```python
from build123d import *

# Parameters (mm, degrees)
SKETCH007_R   = 1.5
SKETCH007_W   = 93.5
SKETCH007_H   = 73
PAD004_DEPTH  = 1.5
SKETCH008_W   = 96.5
SKETCH008_H   = 76
SKETCH008_W_2 = 93.5
SKETCH008_H_2 = 73
PAD005_DEPTH  = 10
FILLET005_R   = 1


with BuildPart() as part:
    # Sketch007 → Pad004 (new body)
    with BuildSketch(Plane.XY):
        with BuildLine():
            Line((-48.25, -33), (-48.25, 33))
            Line((-48.25, 33), (-52.492641, 37.242641))
            ThreePointArc((-47.492641, 42.242641), (-52.492641, 42.242641), (-52.492641, 37.242641))
            Line((-43.25, 38), (-47.492641, 42.242641))
            Line((-43.25, 38), (43.25, 38))
            Line((43.25, 38), (47.492641, 42.242641))
            ThreePointArc((52.492641, 37.242641), (52.492641, 42.242641), (47.492641, 42.242641))
            Line((48.25, 33), (52.492641, 37.242641))
            Line((48.25, 33), (48.25, -33))
            Line((48.25, -33), (52.492641, -37.242641))
            ThreePointArc((47.492641, -42.242641), (52.492641, -42.242641), (52.492641, -37.242641))
            Line((43.25, -38), (47.492641, -42.242641))
            Line((43.25, -38), (-43.25, -38))
            Line((-43.25, -38), (-47.492641, -42.242641))
            ThreePointArc((-52.492641, -37.242641), (-52.492641, -42.242641), (-47.492641, -42.242641))
            Line((-48.25, -33), (-52.492641, -37.242641))
        make_face()
        with Locations((49.992641, -39.742641)):
            Circle(SKETCH007_R, mode=Mode.SUBTRACT)
        with Locations((-49.992641, -39.742641)):
            Circle(SKETCH007_R, mode=Mode.SUBTRACT)
        with Locations((-49.992641, 39.742641)):
            Circle(SKETCH007_R, mode=Mode.SUBTRACT)
        with Locations((49.992641, 39.742641)):
            Circle(SKETCH007_R, mode=Mode.SUBTRACT)
        Rectangle(SKETCH007_W, SKETCH007_H, mode=Mode.SUBTRACT)
    extrude(amount=PAD004_DEPTH)

    # Sketch008 (on Face26 of Pad004) → Pad005 (join)
    with BuildSketch(Plane.XY.offset(1.5)):
        Rectangle(SKETCH008_W, SKETCH008_H)
        Rectangle(SKETCH008_W_2, SKETCH008_H_2, mode=Mode.SUBTRACT)
    extrude(amount=PAD005_DEPTH)

    # Fillet005
    fillet005_edges = [part.edges().sort_by_distance(p)[0] for p in [
        (48.25, -38, 6.5),
        (-48.25, -38, 6.5),
        (48.25, 38, 6.5),
        (-48.25, 38, 6.5),
        (46.75, -36.5, 6.5),
        (-46.75, 36.5, 6.5),
        (46.75, 36.5, 6.5),
        (-46.75, -36.5, 6.5),
    ]]
    fillet(fillet005_edges, radius=FILLET005_R)


with BuildPart() as part_1:
    # Body003 placement: moved
    add(part.part.moved(Location((0, 0, 4.5))))


solid = part_1.part
```
The listing builds one solid part. Answer for the finished solid, in the listing's coordinates (mm). A direction names the side the tool comes from. Give positions to 0.01 mm unless a question says otherwise; leave off trailing zeros. Order: outer loops, then holes, each group sorted by start corner. A loop starts at its lowest first (then second) coordinate and runs counter-clockwise, first axis right, second up. Notation, with made-up numbers: (71, 62.25) -> (107, 62.25) arc R17 cw to (107, 90.25) -> close; hole circle Ø3 at (-6.5, 82.5). An arc over 180 degrees is marked (long way). Answer as a JSON object with one key per item and string values. Group by question number.
Item 1: Consider L1, parallel to X at y = 3, z = 6; L2, parallel to Y at x = 16, z = 5; L3, parallel to X at y = 34, z = 5.5. Determine where each line is inside the solid, lowest interval first. Write a range as from..to.
Item 2: Flat-ended cylindrical pins translate along their axes: pin 1 (2 mm diameter, centred on x = 33.5, z = 6.5, fed in from +Y); pin 2 (1 mm diameter, centred on y = -2, z = 7, fed in from -X); pin 3 (6 mm diameter, centred on x = -18.5, z = 11.5, fed in from -Y). Find the tip coordinate at first contact, or state that the pin passes through.
Item 3: The part is cut by section A-A on y = 6. Write down the section's boundary in (x, z).
Item 4: A tool of negligible diameter and unlimited length cuts with its end or side. For faces 1 (the flat face through (-45.34, 40.09, 5.24)), 2 (the flat face through (46.75, 0, 10)), 3 (the flat face through (48, 39, 6)), 4 (the flat face through (-50.34, 35.09, 5.24)), from which of +Z, -Z, +X, -X, +Y, -Y can it reach the whole face along a straight path? Write none if from no direction.
Item 5: Determine the mould class of faces 5 (the flat face through (-48, -39, 6)), 6 (the cylindrical face through (-52.437, 42.297, 5.24)), 7 (the cylindrical face through (-49.3, 38.41, 5.24)), 8 (the flat face through (50.34, 35.09, 5.24)) for opening direction X: pulls with the +X half, pulls with the -X half, needs draft (parallel to the pull), parting line crosses it, or undercut.
Item 6: The part is cut by section C-C on z = 14.5. Write down the section's boundary in (x, y), and give its area (4 significant figures).
Item 7: The part is cut by section B-B on x = -27.5. Write down the section's boundary in (y, z), and give its area (3 significant figures).
Result set:
{
 "1": {"L1": "-48.25..-46.75, 46.75..48.25", "L2": "-38..-36.5, 36.5..38", "L3": "-49.25..-46.75, 46.75..49.25"},
 "2": {"pin 1": "y = 38", "pin 2": "x = -48.25", "pin 3": "y = -38"},
 "3": {"outline": "(-48.25, 4.5) -> (-46.75, 4.5) -> (-46.75, 16) -> (-48.25, 16) -> close; (46.75, 4.5) -> (48.25, 4.5) -> (48.25, 16) -> (46.75, 16) -> close"},
 "4": {"face 1": "+Z, -Z, +Y", "face 2": "+Z, -Z", "face 3": "+Z, +X, +Y", "face 4": "+Z, -Z, -X"},
 "5": {"face 5": "needs draft", "face 6": "undercut", "face 7": "undercut", "face 8": "pulls with the +X half"},
 "6": {"outline": "(-48.25, -37) arc R1 ccw to (-47.25, -38) -> (47.25, -38) arc R1 ccw to (48.25, -37) -> (48.25, 37) arc R1 ccw to (47.25, 38) -> (-47.25, 38) arc R1 ccw to (-48.25, 37) -> close; hole (-46.75, -35.5) arc R1 ccw to (-45.75, -36.5) -> (45.75, -36.5) arc R1 ccw to (46.75, -35.5) -> (46.75, 35.5) arc R1 ccw to (45.75, 36.5) -> (-45.75, 36.5) arc R1 ccw to (-46.75, 35.5) -> close", "area": "508.5 mm²"},
 "7": {"outline": "(-38, 4.5) -> (-36.5, 4.5) -> (-36.5, 16) -> (-38, 16) -> close; (36.5, 4.5) -> (38, 4.5) -> (38, 16) -> (36.5, 16) -> close", "area": "34.5 mm²"}
}
